For this review, use the dimensioned drawing (mm, ordinates from the lowest corner) and the shaded views. A direction names the side the tool comes from. Give positions to 0.01 mm unless a question says otherwise; leave off trailing zeros. Order: outer loops, then holes, each group sorted by start corner. A loop starts at its lowest first (then second) coordinate and runs counter-clockwise, first axis right, second up. Notation, with made-up numbers: (15.5, 42) - (54.5, 42) arc R27 ccw to (54.5, 78) - close; hole circle Ø3 at (72, 83.25). An arc over 180 degrees is marked (long way). One line per item, written item: value.
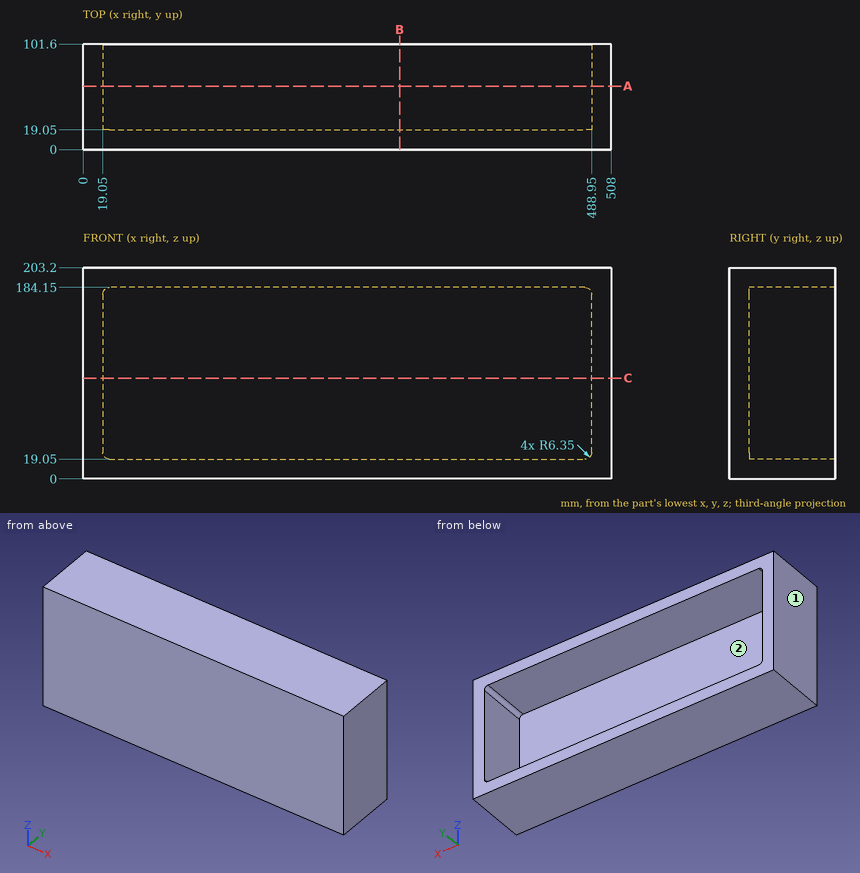
(1) Take a section at B-B (x = 304.5). Write out the cut boundary in (y, z), then the cut area to 3 significant figures.
Answers below:
outline: (0, 0) - (101.6, 0) - (101.6, 19.05) - (19.05, 19.05) - (19.05, 184.15) - (101.6, 184.15) - (101.6, 203.2) - (0, 203.2) - close
area: 7,020 mm^2
(2) Machinability: for the marked faces 1 and 2, which of the approach directions +Z, -Z, +X, -X, +Y, -Y give a long, thin tool a straight path to every point of the face, cutting with its end or side? Answer none if there is none.
Answers below:
face 1: +Z, -Z, -X, +Y, -Y
face 2: +Y
(3) Take a section at A-A (y = 61). Write out the cut boundary in (x, z).
Answers below:
outline: (0, 0) - (508, 0) - (508, 203.2) - (0, 203.2) - close; hole (19.05, 25.4) arc R6.35 ccw to (25.4, 19.05) - (482.6, 19.05) arc R6.35 ccw to (488.95, 25.4) - (488.95, 177.8) arc R6.35 ccw to (482.6, 184.15) - (25.4, 184.15) arc R6.35 ccw to (19.05, 177.8) - close
(4) Wall thickness on line 1 (X direction, y = 54.5, z = 76.5); line 2 (Z direction, x = 419, y = 69); line 3 (Y direction, x = 299.5, z = 176): over which ranges is each line inside the solid? List them lowest first. Write a range as from..to.
Answers below:
line 1: x = 0..19.05, 488.95..508
line 2: z = 0..19.05, 184.15..203.2
line 3: y = 0..19.05
(5) Take a section at C-C (z = 97). Write out the cut boundary in (x, y), then the cut area to 3 significant figures.
Answers below:
outline: (0, 0) - (508, 0) - (508, 101.6) - (488.95, 101.6) - (488.95, 19.05) - (19.05, 19.05) - (19.05, 101.6) - (0, 101.6) - close
area: 12,800 mm^2
